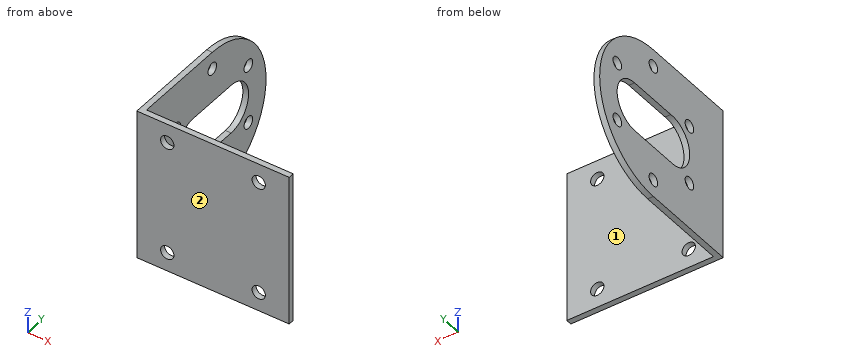
from build123d import *

# Parameters (mm, degrees)
SKETCH_1_W          = 40
SKETCH_1_H          = 40
EXTRUDE_1_DEPTH     = 1.5
SKETCH_4_R          = 1.6
EXTRUDE_2_DEPTH     = 1.5
SKETCH_5_R          = 1.75
CUT_EXTRUDE_1_DEPTH = 1.5


with BuildPart() as part:
    # 草图1 → 凸台-拉伸1 (new body)
    with BuildSketch(Plane(origin=(0, 0, 0), x_dir=(1, 0, 0), z_dir=(0, 1, 0))):
        Rectangle(SKETCH_1_W, SKETCH_1_H)
    extrude(amount=EXTRUDE_1_DEPTH)

    # 草图4 → 凸台-拉伸2 (add)
    with BuildSketch(Plane.ZY.offset(20)):
        with BuildLine():
            Line((-20, 1.5), (20, 1.5))
            Line((20, 1.5), (20, 26))
            ThreePointArc((20, 26), (0, 46), (-20, 26))
            Line((-20, 26), (-20, 1.5))
        make_face()
        with Locations((-7.75, 12.576606241)):
            Circle(SKETCH_4_R, mode=Mode.SUBTRACT)
        with Locations((7.75, 12.576606241)):
            Circle(SKETCH_4_R, mode=Mode.SUBTRACT)
        with Locations((-15.5, 26)):
            Circle(SKETCH_4_R, mode=Mode.SUBTRACT)
        with Locations((-7.75, 39.423393759)):
            Circle(SKETCH_4_R, mode=Mode.SUBTRACT)
        with BuildLine():
            Line((-6.5, 19.528878463), (-6.5, 33))
            ThreePointArc((-6.5, 33), (0, 39.5), (6.5, 33))
            Line((6.5, 33), (6.5, 19.528878463))
            ThreePointArc((6.5, 19.528878463), (0, 12.478519154), (-6.5, 19.528878463))
        make_face(mode=Mode.SUBTRACT)
        with Locations((15.5, 26)):
            Circle(SKETCH_4_R, mode=Mode.SUBTRACT)
        with Locations((7.75, 39.423393759)):
            Circle(SKETCH_4_R, mode=Mode.SUBTRACT)
    extrude(amount=-EXTRUDE_2_DEPTH)

    # 草图5 → 切除-拉伸1 (cut)
    with BuildSketch(Plane(origin=(0, 1.5, 0), x_dir=(1, 0, 0), z_dir=(0, 1, 0))):
        with Locations(Location((12, -15, 0), (0, 0, 270))):
            Circle(SKETCH_5_R)
        with Locations(Location((12, 15, 0), (0, 0, 90))):
            Circle(SKETCH_5_R)
        with Locations(Location((-12, -15, 0), (0, 0, 90))):
            Circle(SKETCH_5_R)
        with Locations(Location((-12, 15, 0), (0, 0, 270))):
            Circle(SKETCH_5_R)
    extrude(amount=-CUT_EXTRUDE_1_DEPTH, mode=Mode.SUBTRACT)


solid = part.part
For this review, take the finished solid that the model builds, in its own axes (mm). Face numbers are marked on the shaded views. A direction names the side the tool comes from. Coordinates: 2 decimals unless noted, no trailing zeros. Write each loop counter-clockwise with the first axis right and the second up, starting at its lowest first coordinate (ties: lowest second). Pieces come first, ordered by that corner, then holes. Notation, with made-up numbers: (2, 58) -> (53, 58) arc R25 ccw to (53, 73) -> close; hole circle Ø1 at (-24, 77.5). An arc over 180 degrees is marked (long way). Write each question's results on one line, items separated by ' | '. Start each with the question number.
1) Consider section D-D (z = 7.75). Write out the cut boundary in (x, y), plus the area to 3 significant figures.
2) Consider section C-C (z = -15.5). Write out the cut boundary in (x, y).
3) Insertion check: pin 1 (5 mm diameter, centred on x = -9.5, z = -8.5, fed in from +Y); pin 2 (6 mm diameter, centred on x = 4.5, z = -6, fed in from -Y); pin 3 (5 mm diameter, centred on y = 39.42, z = 7.75, fed in from +X); pin 4 (0.8 mm diameter, centred on x = -19, y = 27.5, fed in from +Z). Each pin has a flat end and moves straight along its axis. Give the tip position at first contact, or say it passes through.
4) Consider section A-A (x = -12). Write out the cut boundary in (y, z), plus the area to 3 significant figures.
5) Consider section B-B (y = 32). Write out the cut boundary in (x, z).
6) For the marked faces 1 and 2, list the 3-axis set-ups (+Z, -Z, +X, -X, +Y, -Y) from which the entire face can be reached by the end or side of a thin tool; tool diameter is ignored.
7) Wall thickness on L1, parallel to Y at x = -19, z = 0; L2, parallel to X at y = 40.5, z = -11; L3, parallel to Y at x = -18, z = -7: over which ranges is each line inside the solid? List them lowest first. Write a range as [from, to].
Geometry says:
1) outline: (-20, 0) -> (20, 0) -> (20, 1.5) -> (-18.5, 1.5) -> (-18.5, 10.98) -> (-20, 10.98) -> close; (-20, 14.18) -> (-18.5, 14.18) -> (-18.5, 37.82) -> (-20, 37.82) -> close; (-20, 41.02) -> (-18.5, 41.02) -> (-18.5, 44.44) -> (-20, 44.44) -> close | area: 115 mm^2
2) outline: (-20, 0) -> (-13.68, 0) -> (-13.68, 1.5) -> (-18.5, 1.5) -> (-18.5, 24.4) -> (-20, 24.4) -> close; (-20, 27.6) -> (-18.5, 27.6) -> (-18.5, 38.64) -> (-20, 38.64) -> close; (-10.32, 0) -> (10.32, 0) -> (10.32, 1.5) -> (-10.32, 1.5) -> close; (13.68, 0) -> (20, 0) -> (20, 1.5) -> (13.68, 1.5) -> close
3) pin 1: y = 1.5 | pin 2: y = 0 | pin 3: x = -18.5 | pin 4: z = 19.97
4) outline: (0, -20) -> (1.5, -20) -> (1.5, -16.75) -> (0, -16.75) -> close; (0, -13.25) -> (1.5, -13.25) -> (1.5, 13.25) -> (0, 13.25) -> close; (0, 16.75) -> (1.5, 16.75) -> (1.5, 20) -> (0, 20) -> close | area: 49.5 mm^2
5) outline: (-20, -19.08) -> (-18.5, -19.08) -> (-18.5, -6.5) -> (-20, -6.5) -> close; (-20, 6.5) -> (-18.5, 6.5) -> (-18.5, 19.08) -> (-20, 19.08) -> close
6) face 1: +Z, -Z, +X, +Y | face 2: +Z, -Z, +X, -X, -Y
7) L1: [0, 12.48], [39.5, 46] | L2: [-20, -18.5] | L3: [0, 1.5]
